```python
from build123d import *

# Parameters (mm, degrees)
SKETCH1_R                   = 82.55
BOSS_EXTRUDE1_DEPTH         = 10
FILLET1_R                   = 5
F_12_0_189_DIAMETER_HOLE1_D = 4.8006
CIRPATTERN1_COUNT           = 4


with BuildPart() as part:
    # Sketch1 → Boss-Extrude1 (new body)
    with BuildSketch(Plane(origin=(0, 0, 0), x_dir=(1, 0, 0), z_dir=(0, 1, 0))):
        with Locations(Location((0, 0, 0), (0, 0, 270))):
            Circle(SKETCH1_R)
        with BuildLine():
            Line((-42, 52), (-52, 52))
            Line((-52, 52), (-52, 42))
            Line((-52, 42), (-65.192043226, 42))
            ThreePointArc((-65.192043226, 42), (-74.396389201, 21.890175283), (-77.55, 0))
            ThreePointArc((-77.55, 0), (-76.61982896, -11.975153869), (-73.851629653, -23.663036524))
            Line((-73.851629653, -23.663036524), (-69.476634051, -21.85085401))
            ThreePointArc((-69.476634051, -21.85085401), (-61.114631076, -25.314509051), (-64.578286117, -33.676512026))
            Line((-64.578286117, -33.676512026), (-68.953281719, -35.48869454))
            ThreePointArc((-68.953281719, -35.48869454), (-67.151629361, -38.789962286), (-65.192043226, -42))
            Line((-65.192043226, -42), (-52, -42))
            Line((-52, -42), (-52, -52))
            Line((-52, -52), (-42, -52))
            Line((-42, -52), (-42, -65.192043226))
            ThreePointArc((-42, -65.192043226), (-21.890175283, -74.396389201), (0, -77.55))
            ThreePointArc((0, -77.55), (11.975153869, -76.61982896), (23.663036524, -73.851629653))
            Line((23.663036524, -73.851629653), (21.85085401, -69.476634051))
            ThreePointArc((21.85085401, -69.476634051), (25.314509051, -61.114631076), (33.676512026, -64.578286117))
            Line((33.676512026, -64.578286117), (35.48869454, -68.953281719))
            ThreePointArc((35.48869454, -68.953281719), (38.789962286, -67.151629361), (42, -65.192043226))
            Line((42, -65.192043226), (42, -52))
            Line((42, -52), (52, -52))
            Line((52, -52), (52, -42))
            Line((52, -42), (65.192043226, -42))
            ThreePointArc((65.192043226, -42), (74.396389201, -21.890175283), (77.55, 0))
            ThreePointArc((77.55, 0), (76.61982896, 11.975153869), (73.851629653, 23.663036524))
            Line((73.851629653, 23.663036524), (69.476634051, 21.85085401))
            ThreePointArc((69.476634051, 21.85085401), (61.114631076, 25.314509051), (64.578286117, 33.676512026))
            Line((64.578286117, 33.676512026), (68.953281719, 35.48869454))
            ThreePointArc((68.953281719, 35.48869454), (67.151629361, 38.789962286), (65.192043226, 42))
            Line((65.192043226, 42), (52, 42))
            Line((52, 42), (52, 52))
            Line((52, 52), (42, 52))
            Line((42, 52), (42, 65.192043226))
            ThreePointArc((42, 65.192043226), (21.890175283, 74.396389201), (0, 77.55))
            ThreePointArc((0, 77.55), (-11.975153869, 76.61982896), (-23.663036524, 73.851629653))
            Line((-23.663036524, 73.851629653), (-21.85085401, 69.476634051))
            ThreePointArc((-21.85085401, 69.476634051), (-25.314509051, 61.114631076), (-33.676512026, 64.578286117))
            Line((-33.676512026, 64.578286117), (-35.48869454, 68.953281719))
            ThreePointArc((-35.48869454, 68.953281719), (-38.789962286, 67.151629361), (-42, 65.192043226))
            Line((-42, 65.192043226), (-42, 52))
        make_face(mode=Mode.SUBTRACT)
    extrude(amount=BOSS_EXTRUDE1_DEPTH)

    # Fillet1
    # the kernel refuses this fillet: 5 mm, written as the material it adds along each edge
    with BuildSketch(Plane(origin=(-73.851629653, 0, 23.663036524), x_dir=(-0.269371971456704, 0, -0.9630362095962584), z_dir=(0, 1, 0)), Plane(origin=(23.663036524, 0, 73.851629653), x_dir=(-0.9630362095962577, 0, 0.26937197145670677), z_dir=(0, 1, 0)), Plane(origin=(73.851629653, 0, -23.663036524), x_dir=(0.269371971456704, 0, 0.9630362095962584), z_dir=(0, 1, 0)), Plane(origin=(-23.663036524, 0, -73.851629653), x_dir=(0.9630362095962544, 0, -0.26937197145671865), z_dir=(0, 1, 0))) as fillet1_piece_1:
        with BuildLine():
            CenterArc((5.602962852, -4.996515299), FILLET1_R, 87.860754673, 94.506173203)
            Line((0.607228677, -5.203009978), (0.107655259, -5.223659445))
            ThreePointArc((0.107655259, -5.223659445), (0.070289372, -4.761265734), (-0.496406817, -0.059835376))
            Line((-0.496406817, -0.059835376), (-0.0186641, 0.49965153))
            ThreePointArc((-0.0186641, 0.49965153), (2.894801927, 0.554047707), (5.808267953, 0.49965153))
            Line((5.808267953, 0.49965153), (5.789603853, 0))
        make_face()
    extrude(amount=10)
    with BuildSketch(Plane(origin=(-68.953281719, 0, 35.48869454), x_dir=(0.9224276908117425, 0, -0.386169852815722), z_dir=(0, 1, 0)), Plane(origin=(35.48869454, 0, 68.953281719), x_dir=(-0.38616985281572375, 0, -0.9224276908117417), z_dir=(0, 1, 0)), Plane(origin=(68.953281719, 0, -35.48869454), x_dir=(-0.9224276908117431, 0, 0.3861698528157207), z_dir=(0, 1, 0)), Plane(origin=(-35.48869454, 0, -68.953281719), x_dir=(0.3861698528157226, 0, 0.9224276908117423), z_dir=(0, 1, 0))) as fillet1_piece_2:
        with BuildLine():
            CenterArc((5.612329068, -4.985992408), FILLET1_R, 94.289787829, 94.506173203)
            Line((0.67113325, -5.75057327), (0.177013669, -5.827031356))
            ThreePointArc((0.177013669, -5.827031356), (-0.214745972, -2.939512072), (-0.498446682, -0.039381534))
            Line((-0.498446682, -0.039381534), (0.001888314, 0.499996434))
            ThreePointArc((0.001888314, 0.499996434), (4.73731566, 0.482112358), (5.200923615, 0.498599241))
            Line((5.200923615, 0.498599241), (5.238324111, 0))
        make_face()
    extrude(amount=10)
    with BuildSketch(Plane(origin=(-42, 0, 65.192043226), x_dir=(0, 0, -1), z_dir=(0, 1, 0)), Plane(origin=(65.192043226, 0, 42), x_dir=(-1, 0, 0), z_dir=(0, 1, 0)), Plane(origin=(42, 0, -65.192043226), x_dir=(0, 0, 1), z_dir=(0, 1, 0)), Plane(origin=(-65.192043226, 0, -42), x_dir=(1, 0, 0), z_dir=(0, 1, 0))) as fillet1_piece_3:
        with BuildLine():
            CenterArc((2.786093991, -5), FILLET1_R, 90, 59.336629316)
            ThreePointArc((-1.514798445, -2.450034459), (-0.768775648, -1.217983455), (0, 0))
            Line((0, 0), (2.786093991, 0))
        make_face()
    extrude(amount=10)
    with BuildSketch(Plane(origin=(-65.192043226, 0, 42), x_dir=(-0.5258802907220335, 0, -0.8505585928259789), z_dir=(0, 1, 0)), Plane(origin=(42, 0, 65.192043226), x_dir=(-0.8505585928259877, 0, 0.5258802907220195), z_dir=(0, 1, 0)), Plane(origin=(65.192043226, 0, -42), x_dir=(0.5258802907220256, 0, 0.8505585928259839), z_dir=(0, 1, 0))) as fillet1_piece_4:
        with BuildLine():
            CenterArc((2.787641046, -4.999137638), FILLET1_R, 88.935847769, 59.336629316)
            Line((-1.465151918, -2.369736184), (0, 0))
            ThreePointArc((0, 0), (1.440250254, 0.01337524), (2.880500508, 0))
        make_face()
    extrude(amount=10)
    with BuildSketch(Plane(origin=(-42, 0, -65.192043226), x_dir=(0, 0, 1), z_dir=(0, 1, 0))) as fillet1_piece_5:
        with BuildLine():
            CenterArc((2.786093991, 5), FILLET1_R, 210.663370684, 59.336629316)
            ThreePointArc((-1.514798445, 2.450034459), (-0.768775648, 1.217983455), (0, 0))
            Line((0, 0), (2.786093991, 0))
        make_face()
    extrude(amount=10)

    # #12 (0.189) Diameter Hole1 (through all)
    with Locations(Plane(origin=(0, 10, 0), x_dir=(1, 0, 0), z_dir=(0, 1, 0))):
        with Locations((67.027460084, 27.763683018)):
            f_12_0_189_diameter_hole1 = Hole(F_12_0_189_DIAMETER_HOLE1_D / 2)

    # CirPattern1: #12 (0.189) Diameter Hole1 ×4 about axis
    cirpattern1_axis = Axis((0, 0, 0), (0, 1, 0))
    for i in range(1, CIRPATTERN1_COUNT):
        add(f_12_0_189_diameter_hole1.rotate(cirpattern1_axis, i * 360 / CIRPATTERN1_COUNT), mode=Mode.SUBTRACT)


solid = part.part
```
Input: part model. Units: mm. Frame: model coordinates. A direction names the side the tool comes from. Give positions to 0.01 mm unless a question says otherwise; leave off trailing zeros. Order: outer loops, then holes, each group sorted by start corner. A loop starts at its lowest first (then second) coordinate and runs counter-clockwise, first axis right, second up.
1. Line query: probe 1 along Z at (x, y) = (-1, 4); probe 2 along X at (y, z) = (6.25, -56); probe 3 along X at (y, z) = (2.25, 64.5). Output: solid intervals per line, ascending.
Computed:
probe 1: z = -82.54 to -77.54, 77.54 to 82.54
probe 2: x = -60.65 to -42, 42 to 60.65
probe 3: x = -51.52 to -41.54, 21.88 to 33.68, 41.54 to 51.52
2. Cut plane C-C (y = 6.75). State how many separate pieces and enclosed holes the cut face has, and give its area (3 significant figures).
Computed:
separate pieces: 1
enclosed holes: 5
area: 3,850 mm2
3. Draft query along Z for faces 1 (the face through (-25, 0, -62)), 2 (the face through (-67.34, 4.93, 30.144)). Return one class per face: released by +Z, released by -Z, zero draft, split by the parting line, or undercut.
Computed:
face 1: zero draft
face 2: undercut
4. Pin query (flat end, axial travel): pin 1 Ø5 at (y, z) = (7, -48.5) entering from +X; pin 2 Ø5 at (y, z) = (4.5, -59) entering from -X; pin 3 Ø1.5 at (y, z) = (5.5, 31) entering from +X. Return the tip coordinate at first contact, or that it passes through.
Computed:
pin 1: stops at x = 68.55
pin 2: stops at x = -60.19
pin 3: stops at x = 76.81
5. Cut plane B-B (z = -56). Return loops of the section in (x, y), and give its area (3 significant figures).
Computed:
outline: (-60.65, 0) - (-42, 0) - (-42, 10) - (-60.65, 10) - close; (42, 0) - (60.65, 0) - (60.65, 10) - (42, 10) - close
area: 373 mm2
6. Set-up query: faces 3 (the face through (25, 10, 62)), 4 (the face through (64.656, 4.93, -41.465)). Return all of +Z, -Z, +X, -X, +Y, -Y with unobstructed straight access to the full face (end or side cutting, diameter ignored); none if empty.
Computed:
face 3: +Z, -Z, +X, -X, +Y
face 4: +Y, -Y
7. Cut plane A-A (z = 5). Return loops of the section in (x, y), and give its area (3 significant figures).
Computed:
outline: (-82.4, 0) - (-77.39, 0) - (-77.39, 10) - (-82.4, 10) - close; (77.39, 0) - (82.4, 0) - (82.4, 10) - (77.39, 10) - close
area: 100 mm2
